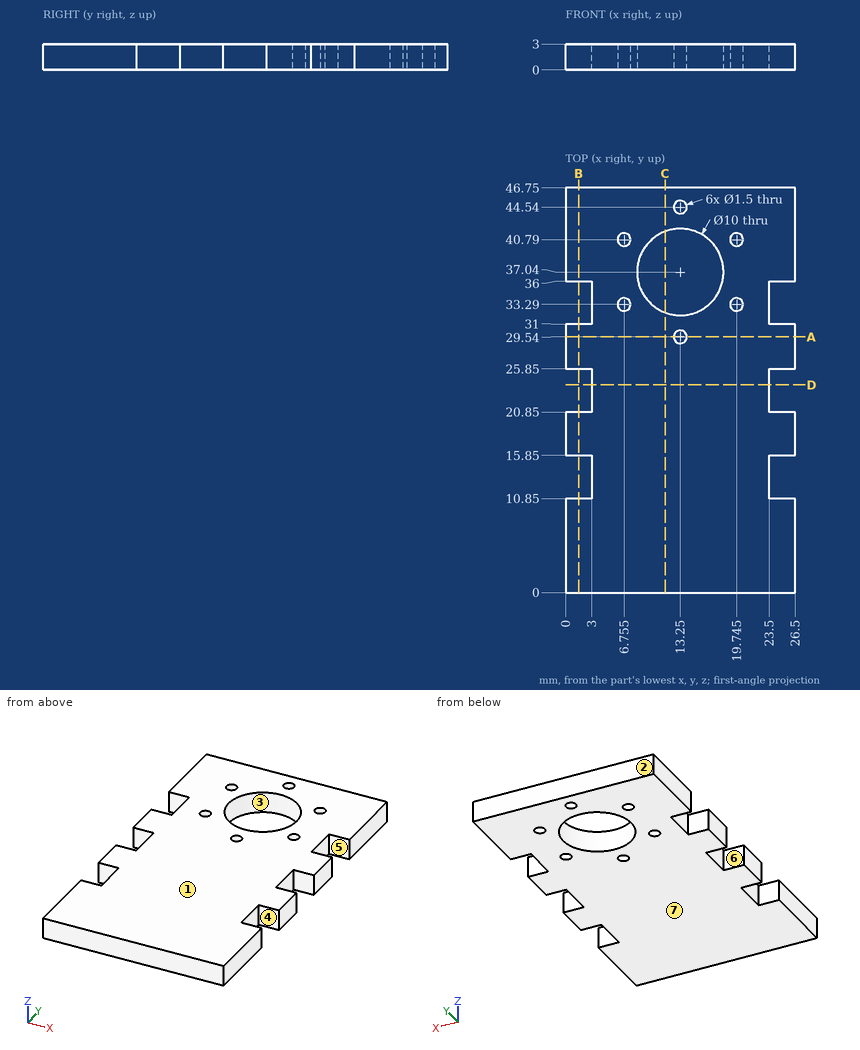
Input: dimensioned drawing with shaded views. Units: mm. Origin: part minimum x, y, z. A direction names the side the tool comes from. Give positions to 0.01 mm unless a question says otherwise; leave off trailing zeros. Write each loop counter-clockwise with the first axis right and the second up, starting at its lowest first coordinate (ties: lowest second). Pieces come first, ordered by that corner, then holes. Notation, with made-up numbers: M -23.75,-16 L -2.75,-16 A33 cw -2.75,15 Z; hole C 75,28 d8. An arc over 180 degrees is marked long. Write item = value, one per line. Start each with the question number.
1) Draft query along Y for the marked faces 1, 2, 3 and 4. Return one class per face: +Y half, -Y half, draft (parallel to the pull), parting line (faces both ways), or undercut.
2) Material intervals for line 1 along Y through (x, z) = (24, 2.25); line 2 along Y through (x, z) = (13.25, 1.9); line 3 along X through (y, z) = (44.5, 1.5), sorted ascending. Write a range as [from, to].
3) Cut plane B-B on x = 1.5. Return the cut outline in (y, z).
4) Cut plane C-C on x = 11.5. Return the cut outline in (y, z), then the cut area to 3 significant figures.
5) Reachability of the marked faces 5, 6 and 7 from +Z, -Z, +X, -X, +Y, -Y: full face, straight path, thin tool, end or side. Return the list, or none.
6) Cut plane A-A on y = 29.54. Return the cut outline in (x, z), then the cut area to 3 significant figures.
7) Cut plane D-D on y = 24. Return the cut outline in (x, z).
8) First-contact query: pin 1 Ø1.2 at (x, y) = (13.25, 44.54) entering from -Z; pin 2 Ø1.5 at (y, z) = (34.5, 1.5) entering from -X; pin 3 Ø0.9 at (y, z) = (14, 1.5) entering from +X. Flat tips, straight axial feed; report the tip coordinate or a pass-through.
Solved:
q1.face_1 = draft
q1.face_2 = +Y half
q1.face_3 = undercut
q1.face_4 = undercut
q2.line_1 = [0, 10.85], [15.85, 20.85], [25.85, 31], [36, 46.75]
q2.line_2 = [0, 28.79], [30.29, 32.04], [42.04, 43.79], [45.29, 46.75]
q2.line_3 = [0, 12.5], [14, 26.5]
q3.outline = M 0,0 L 10.85,0 L 10.85,3 L 0,3 Z; M 15.85,0 L 20.85,0 L 20.85,3 L 15.85,3 Z; M 25.85,0 L 31,0 L 31,3 L 25.85,3 Z; M 36,0 L 46.75,0 L 46.75,3 L 36,3 Z
q4.outline = M 0,0 L 32.36,0 L 32.36,3 L 0,3 Z; M 41.72,0 L 46.75,0 L 46.75,3 L 41.72,3 Z
q4.area = 112 mm2
q5.face_5 = +Z, -Z, +X
q5.face_6 = +Z, -Z, -X
q5.face_7 = -Z, +X, -X, +Y, -Y
q6.outline = M 0,0 L 12.5,0 L 12.5,3 L 0,3 Z; M 14,0 L 26.5,0 L 26.5,3 L 14,3 Z
q6.area = 75.0 mm2
q7.outline = M 3,0 L 23.5,0 L 23.5,3 L 3,3 Z
q8.pin_1 = through
q8.pin_2 = 3
q8.pin_3 = 23.5
